from build123d import *

# Parameters (mm, degrees)
F1_DEPTH = 6
F3_DEPTH = 4
F4_R     = 0.5
F5_DEPTH = 3
F6_R     = 0.5
F7_DEPTH = 12.9


with BuildPart() as f1:
    # F0 (on Top) → F1 (new body)
    with BuildSketch(Plane.XY):
        with BuildLine():
            Line((4, 1), (1.7320508076, 1))
            ThreePointArc((1.7320508076, 1), (1, 1.7320508076), (0, 2))
            ThreePointArc((0, 2), (-1, 1.7320508076), (-1.7320508076, 1))
            Line((-1.7320508076, 1), (-4, 1))
            Line((-4, 1), (-4, 3))
            Line((-4, 3), (-6.9135528726, 3))
            ThreePointArc((-6.9135528726, 3), (-9, 0), (-6.9135528726, -3))
            Line((-6.9135528726, -3), (-4, -3))
            Line((-4, -3), (-4, -1))
            Line((-4, -1), (-1.7320508076, -1))
            ThreePointArc((-1.7320508076, -1), (-1, -1.7320508076), (0, -2))
            ThreePointArc((0, -2), (1, -1.7320508076), (1.7320508076, -1))
            Line((1.7320508076, -1), (4, -1))
            Line((4, -1), (4, -3))
            Line((4, -3), (6.9135528726, -3))
            ThreePointArc((6.9135528726, -3), (9, 0), (6.9135528726, 3))
            Line((6.9135528726, 3), (4, 3))
            Line((4, 3), (4, 1))
        make_face()
    extrude(amount=F1_DEPTH)

    # F2 (on face) → F3 (cut)
    with BuildSketch(Plane(origin=(0, 0, 0), x_dir=(1, 0, 0), z_dir=(0, 0, -1))):
        with BuildLine():
            ThreePointArc((-1.7320508076, -1), (-2, 0), (-1.7320508076, 1))
            Line((-1.7320508076, 1), (-4, 1))
            Line((-4, 1), (-4, -1))
            Line((-4, -1), (-1.7320508076, -1))
        make_face()
        with BuildLine():
            ThreePointArc((1.7320508076, 1), (2, 0), (1.7320508076, -1))
            Line((1.7320508076, -1), (4, -1))
            Line((4, -1), (4, 1))
            Line((4, 1), (1.7320508076, 1))
        make_face()
    extrude(amount=-F3_DEPTH, mode=Mode.SUBTRACT)

    # F4 (on face) → F5 (join)
    with BuildSketch(Plane.XY.offset(6)):
        Circle(F4_R)
    extrude(amount=F5_DEPTH)

    # F6 (on face) → F7 (join)
    with BuildSketch(Plane(origin=(0, 0, 0), x_dir=(1, 0, 0), z_dir=(0, 0, -1))):
        Circle(F6_R)
    extrude(amount=F7_DEPTH)


solid = f1.part
The listing builds one solid part. Answer for the finished solid, in the listing's coordinates (mm). A direction names the side the tool comes from. Give positions to 0.01 mm unless a question says otherwise; leave off trailing zeros. Loops run counter-clockwise (first coordinate to the right, second up) from the corner with the lowest first, then second, coordinate; pieces in that order, holes last. Notation, with made-up numbers: (86, 14) - (101, 14) arc R15 ccw to (101, 40) - close; hole circle Ø5 at (59.5, 74.25). An arc over 180 degrees is marked (long way). Answer as a JSON object with one key per item and string values.
1. Flat-ended cylindrical pins translate along their axes: pin 1 Ø1.6 at (x, y) = (3, -0.5) entering from -Z; pin 2 Ø0.6 at (x, z) = (-2.5, 5) entering from -Y; pin 3 Ø1 at (x, z) = (3, 5) entering from +Y. Find the tip coordinate at first contact, or state that the pin passes through.
Determined:
{"pin 1": "z = 4", "pin 2": "y = -1", "pin 3": "y = 1"}
2. A cutting plane is placed at B-B (y = 0). Write down the section's boundary in (x, z), then the cut area to 3 significant figures.
Determined:
{"outline": "(-9, 0) - (-4, 0) - (-4, 4) - (-2, 4) - (-2, 0) - (-0.5, 0) - (-0.5, -12.9) - (0.5, -12.9) - (0.5, 0) - (2, 0) - (2, 4) - (4, 4) - (4, 0) - (9, 0) - (9, 6) - (0.5, 6) - (0.5, 9) - (-0.5, 9) - (-0.5, 6) - (-9, 6) - close", "area": "108 mm²"}
3. A cutting plane is placed at A-A (z = 3.5). Write down the section's boundary in (x, y).
Determined:
{"outline": "(-6.91, -3) - (-4, -3) - (-4, 3) - (-6.91, 3) arc R3.2 ccw to start; circle Ø4 at (0, 0); (4, -3) - (6.91, -3) arc R3.2 ccw to (6.91, 3) - (4, 3) - close"}
4. For a pull along X with two mould halves and no side action, classify faces 1 (the cylindrical face through (-0.108, -0.488, 7.479)), 2 (the flat face through (0, 0, 9)), 3 (the flat face through (3, 1, 5)) as pulls with the +X half, pulls with the -X half, needs draft (parallel to the pull), parting line crosses it, or undercut.
Determined:
{"face 1": "parting line crosses it", "face 2": "needs draft", "face 3": "undercut"}
5. Find the intervals of material crossed by L1, parallel to X at y = -1.25, z = 3.25; L2, parallel to Z at x = 4.5, y = 2.25; L3, parallel to X at y = 1, z = 1, in increasing order. Write a range as [from, to].
Determined:
{"L1": "[-8.75, -4], [-1.56, 1.56], [4, 8.75]", "L2": "[0, 6]", "L3": "[-8.84, -4], [-1.73, 1.73], [4, 8.84]"}
6. A cutting plane is placed at C-C (y = -1.25). Write down the section's boundary in (x, z).
Determined:
{"outline": "(-8.75, 0) - (-4, 0) - (-4, 6) - (-8.75, 6) - close; (-1.56, 0) - (1.56, 0) - (1.56, 6) - (-1.56, 6) - close; (4, 0) - (8.75, 0) - (8.75, 6) - (4, 6) - close"}
7. For faces 4 (the flat face through (-3, -1, 5)), 5 (the flat face through (-7, 0, 0)), 6 (the flat face through (6, 0, 0)), determine the directions among +Z, -Z, +X, -X, +Y, -Y from which every point of the face is accessible in a straight line to the end or side of a thin tool.
Determined:
{"face 4": "+Z, -Z, -Y", "face 5": "-Z, -X, +Y, -Y", "face 6": "-Z, +X, +Y, -Y"}
8. A cutting plane is placed at D-D (x = -5.5). Write down the section's boundary in (y, z).
Determined:
{"outline": "(-3, 0) - (3, 0) - (3, 6) - (-3, 6) - close"}
